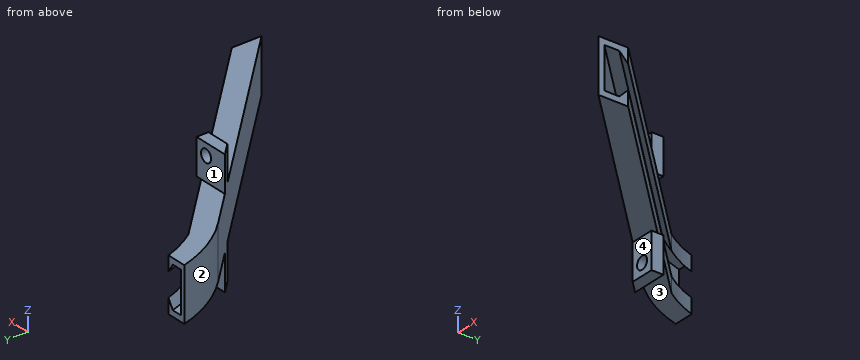
```python
from build123d import *

# Parameters (mm, degrees)
CUT_EXTRUDE1_DEPTH      = 210.179727901
BOSS_EXTRUDE3_DEPTH     = 19.05
F_1_4_CLEARANCE_HOLE1_D = 6.7564


with BuildPart() as part:
    # Sweep1: sweep along a path in Sketch1
    with BuildLine(Plane.XY) as sweep1_path:
        Line((0, 0), (-112.58934785, 112.58934785))
        ThreePointArc((-112.58934785, 112.58934785), (-124.451195327, 128.04800845), (-131.907864376, 146.05))
    # Sketch2 → Sweep1 (sweep)
    with BuildSketch(Plane(origin=(0, 0, 0), x_dir=(0, 0, -1), z_dir=(1, 0, 0))):
        Polygon((0, 0), (14.175, 0), (14.175, 15.9375), (6.2375, 15.9375), (11, 11.175), (11, 3.175), (-11, 3.175), (-11, 11.175), (-6.2375, 15.9375), (-14.175, 15.9375), (-14.175, 0), align=None)
    sweep(path=sweep1_path.line)

    # Sketch3 → Cut-Extrude1 (cut, through all)
    with BuildSketch(Plane(origin=(0, 0, 14.175), x_dir=(-1, 0, 0), z_dir=(0, 0, -1))):
        Polygon((131.907864376, 146.05), (121.208421138, 146.05), (123.939114376, 159.852279873), align=None)
    extrude(amount=CUT_EXTRUDE1_DEPTH, mode=Mode.SUBTRACT)

    # Sketch10 → Boss-Extrude3 (add)
    with BuildSketch(Plane.XY.offset(14.175)):
        Polygon((-88.9, 88.9), (-95.25, 95.25), (-76.2, 95.25), (-76.2, 88.9), align=None)
    boss_extrude3 = extrude(amount=BOSS_EXTRUDE3_DEPTH)

    # 1/4 Clearance Hole1 (through all)
    with Locations(Plane(origin=(0, 95.25, 0), x_dir=(1, 0, 0), z_dir=(0, 1, 0))):
        with Locations((-82.55, -26.875)):
            f_1_4_clearance_hole1 = Hole(F_1_4_CLEARANCE_HOLE1_D / 2)

    # Mirror1: Boss-Extrude3, 1/4 Clearance Hole1 across plane
    add(boss_extrude3.mirror(Plane.XY))
    add(f_1_4_clearance_hole1.mirror(Plane.XY), mode=Mode.SUBTRACT)


solid = part.part
```
Here's how the part is built. I have some questions about the finished solid (model axes, mm). Face numbers are marked on the shaded views. A direction names the side the tool comes from. Round coordinates to 2 decimals unless told otherwise and drop trailing zeros. Loops run counter-clockwise (first coordinate to the right, second up) from the corner with the lowest first, then second, coordinate; pieces in that order, holes last. Notation, with made-up numbers: (3.25, -2) -> (42.25, -2) arc R5 ccw to (42.25, 4) -> close; hole circle Ø6 at (73, 73.5). An arc over 180 degrees is marked (long way). Answer as CSV lines item,"result". Start each with the question number.
1. Imagine slicing it at A-A on x = -82.55. State how many separate pieces and enclosed holes the cut face has, plus the area to 3 significant figures.
2. Imagine slicing it at B-B on x = -106. Write out the boundary of the cut face in (y, z) (1 decimal).
3. I need wall thicknesses on probe 1 along Z at (x, y) = (-82.55, 91.25) (3 decimals); probe 2 along Z at (x, y) = (-82, 94) (3 decimals); probe 3 along Z at (x, y) = (-106, 114) (3 decimals). Which ranges of each line are inside material? Lowest first, please. Write a range as from..to.
4. Imagine slicing it at D-D on y = 66. Write out the boundary of the cut face in (x, z) (1 decimal), plus the area to 3 significant figures.
5. Imagine slicing it at C-C on z = 16.5. Write out the boundary of the cut face in (x, y), plus the area to 3 significant figures.
6. I'm going to push flat-ended pins straight in: P1, Ø6, axis at y = 81.5, z = -7.5, coming from the -X side; P2, Ø1.9, axis at y = 91.5, z = 22.5, coming from the +X side; P3, Ø10, axis at y = 21.5, z = -15.5, coming from the -X side. Where does each tip first touch, or does it pass through?
7. For the marked faces 1, 2, 3 and 4, which set-ups out of +Z, -Z, +X, -X, +Y, -Y let a thin tool reach every point of the face, with its end or its side?
Solution:
1,separate pieces,"3"
1,enclosed holes,"0"
1,area,"350 mm²"
2,outline,"(106, -14.2) -> (121.9, -14.2) -> (121.9, -6.2) -> (117.2, -11) -> (109.2, -11) -> (109.2, 11) -> (117.2, 11) -> (121.9, 6.2) -> (121.9, 14.2) -> (106, 14.2) -> close"
3,probe 1,"-33.225..-30.253, -23.497..-11, 11..23.497, 30.253..33.225"
3,probe 2,"-33.225..-30.208, -23.542..-10.175, 10.175..23.542, 30.208..33.225"
3,probe 3,"-14.175..-11, 11..14.175"
4,outline,"(-66, -14.2) -> (-50.1, -14.2) -> (-50.1, -6.2) -> (-54.8, -11) -> (-62.8, -11) -> (-62.8, 11) -> (-54.8, 11) -> (-50.1, 6.2) -> (-50.1, 14.2) -> (-66, 14.2) -> close"
4,area,"194 mm²"
5,outline,"(-95.25, 95.25) -> (-88.9, 88.9) -> (-76.2, 88.9) -> (-76.2, 95.25) -> close"
5,area,"101 mm²"
6,P1,"x = -84.5"
6,P2,"x = -76.2"
6,P3,"x = -26.32"
7,face 1,"+Z, +X, -X, +Y"
7,face 2,"+Z, -Z, -X, -Y"
7,face 3,"-Z, +X, -X, +Y"
7,face 4,"-Z, +X, -X, -Y"
